Part model, mm, in its own coordinate system. Give positions to 0.01 mm unless a question says otherwise; leave off trailing zeros. Loops run counter-clockwise (first coordinate to the right, second up) from the corner with the lowest first, then second, coordinate; pieces in that order, holes last. Notation, with made-up numbers: (65, 82) -> (115, 82) arc R20 ccw to (115, 87) -> close; hole circle Ø7 at (-11, 61.25). An arc over 180 degrees is marked (long way). Write item = value, one per line.
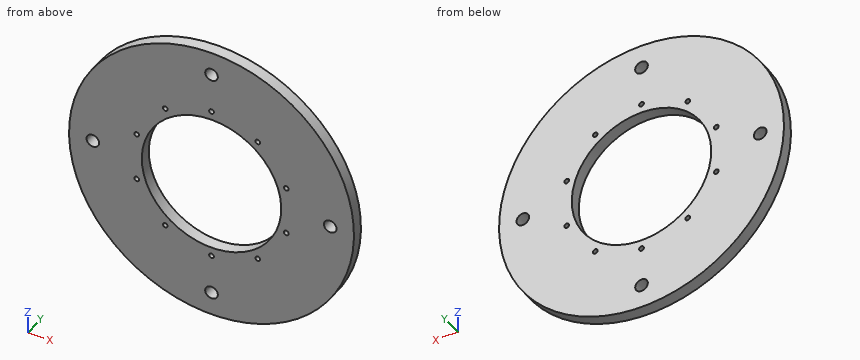
from build123d import *

# Parameters (mm, degrees)
SKETCH1_R                           = 152.4
SKETCH1_R_2                         = 74.6125
THRUSTPLATE_TC3_DEPTH               = 12.7
UNDEF_CLEARANCE_THRUSTPLATE_D       = 13.49248
CLEARANCE_THRUSTPLATE_PATTERN_COUNT = 4
F_10_CLEARANCE_HOLE1_D              = 5.1054
CIRPATTERN1_COUNT                   = 10


with BuildPart() as part:
    # Sketch1 → ThrustPlate_TC3 (new body)
    with BuildSketch(Plane(origin=(0, 0, 0), x_dir=(1, 0, 0), z_dir=(0, 1, 0))):
        with Locations(Location((0, 0, 0), (0, 0, 270))):
            Circle(SKETCH1_R)
        with Locations(Location((0, 0, 0), (0, 0, 270))):
            Circle(SKETCH1_R_2, mode=Mode.SUBTRACT)
    extrude(amount=-THRUSTPLATE_TC3_DEPTH)

    # UNDEF_Clearance_ThrustPlate (through all)
    with Locations(Plane(origin=(0, 0, 0), x_dir=(1, 0, 0), z_dir=(0, 1, 0))):
        with Locations((0, 127)):
            undef_clearance_thrustplate = Hole(UNDEF_CLEARANCE_THRUSTPLATE_D / 2)

    # Clearance_ThrustPlate_Pattern: UNDEF_Clearance_ThrustPlate ×4 about axis
    clearance_thrustplate_pattern_axis = Axis((0, 0, 0), (0, 1, 0))
    for i in range(1, CLEARANCE_THRUSTPLATE_PATTERN_COUNT):
        add(undef_clearance_thrustplate.rotate(clearance_thrustplate_pattern_axis, i * 360 / CLEARANCE_THRUSTPLATE_PATTERN_COUNT), mode=Mode.SUBTRACT)

    # #10 Clearance Hole1 (through all)
    with Locations(Plane(origin=(0, 0, 0), x_dir=(1, 0, 0), z_dir=(0, 1, 0))):
        with Locations((0, 84.1375)):
            f_10_clearance_hole1 = Hole(F_10_CLEARANCE_HOLE1_D / 2)

    # CirPattern1: #10 Clearance Hole1 ×10 about axis
    cirpattern1_axis = Axis((0, 0, 0), (0, 1, 0))
    for i in range(1, CIRPATTERN1_COUNT):
        add(f_10_clearance_hole1.rotate(cirpattern1_axis, i * 360 / CIRPATTERN1_COUNT), mode=Mode.SUBTRACT)


solid = part.part
1) Slice it at A-A, the plane z = 0. List the corners of the cut face in (x, y), and give its area (3 significant figures).
Resolved:
outline = (-152.4, -12.7) -> (-133.75, -12.7) -> (-133.75, 0) -> (-152.4, 0) -> close; (-120.25, -12.7) -> (-74.61, -12.7) -> (-74.61, 0) -> (-120.25, 0) -> close; (74.61, -12.7) -> (120.25, -12.7) -> (120.25, 0) -> (74.61, 0) -> close; (133.75, -12.7) -> (152.4, -12.7) -> (152.4, 0) -> (133.75, 0) -> close
area = 1,630 mm²
2) Slice it at C-C, the plane y = -8.25. Count the separate pieces of the cut face and the enclosed holes in it, and give its area (3 significant figures).
Resolved:
separate_pieces = 1
enclosed_holes = 15
area = 54,700 mm²
3) Slice it at D-D, the plane z = 127. List the corners of the cut face in (x, y), and give its area (3 significant figures).
Resolved:
outline = (-84.24, -12.7) -> (-6.75, -12.7) -> (-6.75, 0) -> (-84.24, 0) -> close; (6.75, -12.7) -> (84.24, -12.7) -> (84.24, 0) -> (6.75, 0) -> close
area = 1,970 mm²
4) Drill centre lines: line 1 along X through (y, z) = (-7.25, 0); line 2 along X through (y, z) = (-9.75, 67); line 3 along Z through (x, y) = (132.5, -9.5). Where is each one in solid material? Low to high. Write a range as [from, to].
Resolved:
line_1 = [-152.4, -133.75], [-120.25, -74.61], [74.61, 120.25], [133.75, 152.4]
line_2 = [-136.88, -51.77], [-47.14, -32.83], [32.83, 47.14], [51.77, 136.88]
line_3 = [-75.3, -3.91], [3.91, 75.3]
5) Slice it at B-B, the plane x = 27. List the corners of the cut face in (y, z).
Resolved:
outline = (-12.7, -149.99) -> (0, -149.99) -> (0, -69.56) -> (-12.7, -69.56) -> close; (-12.7, 69.56) -> (0, 69.56) -> (0, 149.99) -> (-12.7, 149.99) -> close
6) Drop flat-ended pins along their axis: P1, Ø21.5, axis at x = 0, z = -127, coming from the -Y side; P2, Ø1.5, axis at x = -66.5, y = -10.5, coming from the -Z side; P3, Ø1.5, axis at y = -10, z = 29.5, coming from the -X side; P4, Ø4, axis at x = -65.5, y = -4, coming from the +Z side. Give the stop position or say it passes through.
Resolved:
P1 = -12.7
P2 = -137.49
P3 = -149.66
P4 = 138.54
